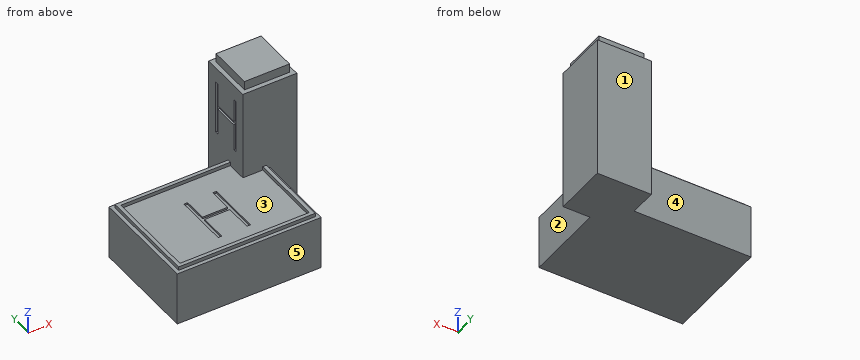
```python
from build123d import *

# Parameters (mm, degrees)
F0_W      = 19.05
F0_H      = 19.05
F1_DEPTH  = 38.1
F2_DEPTH  = 101.6
F3_W      = 31.75
F3_H      = 31.75
F4_DEPTH  = 6.35
F5_W      = 17.78
F5_H      = 2.54
F6_DEPTH  = 1.27
F7_W      = 77.4077631491
F7_H      = 2.54
F7_W_2    = 2.54
F7_H_2    = 52.07
F8_DEPTH  = 2.54
F9_W      = 17.78
F9_H      = 2.54
F10_DEPTH = 1.27


with BuildPart() as f1:
    # F0 (on Top) → F1 (new body)
    with BuildSketch(Plane.XY):
        Polygon((31.75, 38.1), (-50.8, 38.1), (-50.8, -38.1), (50.8, -38.1), (50.8, 19.05), (31.75, 19.05), align=None)
        with Locations((41.275, 28.575)):
            Rectangle(F0_W, F0_H)
    extrude(amount=F1_DEPTH)

    # F0 (on Top) → F2 (join)
    with BuildSketch(Plane.XY):
        Polygon((31.75, 57.15), (31.75, 38.1), (50.8, 38.1), (50.8, 19.05), (69.85, 19.05), (69.85, 57.15), align=None)
        with Locations((41.275, 28.575)):
            Rectangle(F0_W, F0_H)
    extrude(amount=F2_DEPTH)

    # F3 (on face) → F4 (join)
    with BuildSketch(Plane.XY.offset(101.6)):
        with Locations((50.8, 38.1)):
            Rectangle(F3_W, F3_H)
    extrude(amount=F4_DEPTH)

    # F5 (on face) → F6 (cut)
    with BuildSketch(Plane.XY.offset(38.1)):
        with Locations((0, -1.27)):
            Rectangle(F5_W, F5_H)
        Polygon((-8.89, 16.51), (-11.43, 16.51), (-11.43, -21.59), (-8.89, -21.59), (-8.89, -2.54), (-8.89, 0), align=None)
        Polygon((11.43, -21.59), (11.43, 16.51), (8.89, 16.51), (8.89, 0), (8.89, -2.54), (8.89, -21.59), align=None)
    extrude(amount=-F6_DEPTH, mode=Mode.SUBTRACT)

    # F7 (on face) → F8 (join)
    with BuildSketch(Plane.XY.offset(38.1)):
        with Locations((-6.9538815746, 34.29)):
            Rectangle(F7_W, F7_H)
        Polygon((-45.6577631491, 35.56), (-48.1977631491, 35.56), (-48.1977631491, -35.56), (-45.6577631491, -35.56), (-45.6577631491, -33.02), (-45.6577631491, 33.02), align=None)
        Polygon((-45.6577631491, -33.02), (-45.6577631491, -35.56), (48.3222368509, -35.56), (48.3222368509, -33.02), (45.7822368509, -33.02), align=None)
        with Locations((47.0522368509, -6.985)):
            Rectangle(F7_W_2, F7_H_2)
    extrude(amount=F8_DEPTH)

    # F9 (on face) → F10 (cut)
    with BuildSketch(Plane(origin=(31.75, 0, 0), x_dir=(0, -1, 0), z_dir=(-1, 0, 0))):
        Polygon((-46.99, 90.7755655977), (-49.53, 90.7755655977), (-49.53, 52.6755655977), (-46.99, 52.6755655977), (-46.99, 71.7255655977), (-46.99, 74.2655655977), align=None)
        with Locations((-38.1, 72.9955655977)):
            Rectangle(F9_W, F9_H)
        Polygon((-29.21, 90.7755655977), (-29.21, 74.2655655977), (-29.21, 71.7255655977), (-29.21, 52.6755655977), (-26.67, 52.6755655977), (-26.67, 90.7755655977), align=None)
    extrude(amount=-F10_DEPTH, mode=Mode.SUBTRACT)


solid = f1.part
```
Work out the finished part from the listing and answer in its coordinate system (mm). Face numbers are marked on the shaded views. A direction names the side the tool comes from. Coordinates: 2 decimals unless noted, no trailing zeros. Loops run counter-clockwise (first coordinate to the right, second up) from the corner with the lowest first, then second, coordinate; pieces in that order, holes last. Notation, with made-up numbers: (18, 31.25) - (49, 31.25) arc R22 ccw to (49, 47.25) - close; hole circle Ø7 at (20.25, 58). An arc over 180 degrees is marked (long way). Use a Markdown table: item, result.
Item 1: Find section A-A, the plane x = -43.5. Determine the outline of the cut face in (y, z).
Evaluation:
| item | result |
|---|---|
| outline | (-38.1, 0) - (38.1, 0) - (38.1, 38.1) - (35.56, 38.1) - (35.56, 40.64) - (33.02, 40.64) - (33.02, 38.1) - (-33.02, 38.1) - (-33.02, 40.64) - (-35.56, 40.64) - (-35.56, 38.1) - (-38.1, 38.1) - close |
Item 2: Find section C-C, the plane y = -10. Determine the outline of the cut face in (x, z).
Evaluation:
| item | result |
|---|---|
| outline | (-50.8, 0) - (50.8, 0) - (50.8, 38.1) - (48.32, 38.1) - (48.32, 40.64) - (45.78, 40.64) - (45.78, 38.1) - (11.43, 38.1) - (11.43, 36.83) - (8.89, 36.83) - (8.89, 38.1) - (-8.89, 38.1) - (-8.89, 36.83) - (-11.43, 36.83) - (-11.43, 38.1) - (-45.66, 38.1) - (-45.66, 40.64) - (-48.2, 40.64) - (-48.2, 38.1) - (-50.8, 38.1) - close |
Item 3: Find section B-B, the plane z = 23. Determine the outline of the cut face in (x, y).
Evaluation:
| item | result |
|---|---|
| outline | (-50.8, -38.1) - (50.8, -38.1) - (50.8, 19.05) - (69.85, 19.05) - (69.85, 57.15) - (31.75, 57.15) - (31.75, 38.1) - (-50.8, 38.1) - close |
Item 4: Given pin 1 Ø12 at (x, z) = (-6.5, 44.5) entering from -Y; pin 2 Ø1.5 at (x, y) = (36.5, 5.5) entering from +Z; pin 3 Ø1.3 at (y, z) = (-8.5, 39.5) entering from -X, each flat-ended and moving along its own axis, determine where each tip first touches the part or whether it passes through.
Evaluation:
| item | result |
|---|---|
| pin 1 | stops at y = -35.56 |
| pin 2 | stops at z = 38.1 |
| pin 3 | stops at x = -48.2 |
Item 5: The mould has two halves that part along Y. Classify the marked faces 1, 2 and 3: +Y half, -Y half, draft (parallel to the pull), parting line (faces both ways), or undercut.
Evaluation:
| item | result |
|---|---|
| face 1 | +Y half |
| face 2 | draft |
| face 3 | undercut |
Item 6: Consider probe 1 along X at (y, z) = (53, 72); probe 2 along X at (y, z) = (28.5, 69); probe 3 along Z at (x, y) = (-43.5, 1). Determine where each line is inside the solid, lowest interval first. Write a range as from..to.
Evaluation:
| item | result |
|---|---|
| probe 1 | x = 31.75..69.85 |
| probe 2 | x = 33.02..69.85 |
| probe 3 | z = 0..38.1 |
Item 7: Find section D-D, the plane x = 54. Determine the outline of the cut face in (y, z) (3 decimals), and give its area (3 significant figures).
Evaluation:
| item | result |
|---|---|
| outline | (19.05, 0) - (57.15, 0) - (57.15, 101.6) - (53.975, 101.6) - (53.975, 107.95) - (22.225, 107.95) - (22.225, 101.6) - (19.05, 101.6) - close |
| area | 4,070 mm2 |
Item 8: For the marked faces 4 and 5, determine the directions among +Z, -Z, +X, -X, +Y, -Y from which every point of the face is accessible in a straight line to the end or side of a thin tool.
Evaluation:
| item | result |
|---|---|
| face 4 | +Z, -Z, -X, +Y |
| face 5 | +Z, -Z, +X, -X, -Y |
